```python
from build123d import *

# Parameters (mm, degrees)
ESQUISSE3_W                  = 50
ESQUISSE3_H                  = 43
BOSS_EXTRU_1_DEPTH           = 9
ESQUISSE4_R                  = 2.5
ENL_V_MAT_EXTRU_1_DEPTH      = 1
ENL_V_MAT_EXTRU_1_DEPTH_BACK = 10


with BuildPart() as part:
    # Esquisse3 → Boss.-Extru.1 (new body)
    with BuildSketch(Plane.XY):
        with Locations((25, 21.5)):
            Rectangle(ESQUISSE3_W, ESQUISSE3_H)
    extrude(amount=BOSS_EXTRU_1_DEPTH)

    # Esquisse4 → Enlèv. mat.-Extru.1 (cut, two sides)
    with BuildSketch(Plane.XY.offset(9)) as enl_v_mat_extru_1_sk:
        with Locations((25, 21.5)):
            Circle(ESQUISSE4_R)
    extrude(amount=ENL_V_MAT_EXTRU_1_DEPTH, mode=Mode.SUBTRACT)
    extrude(enl_v_mat_extru_1_sk.sketch, amount=-ENL_V_MAT_EXTRU_1_DEPTH_BACK, mode=Mode.SUBTRACT)


solid = part.part
```
Geometry check sheet. Reference: the model listing, model coordinates, mm. Coordinates: 2 decimals unless noted, no trailing zeros. Order: outer loops, then holes, each group sorted by start corner. A loop starts at its lowest first (then second) coordinate and runs counter-clockwise, first axis right, second up.
Item 1: Mould release check, pull along Y, two halves, no side actions. Record for faces 1 (the cylindrical face through (25, 24, 5)), 2 (the flat face through (25, 43, 4)), 3 (the flat face through (25, 0, 4)), 4 (the flat face through (25, 27, 0)): released by +Y, released by -Y, zero draft, split by the parting line, or undercut.
Item 2: Section check A-A (y = 21.5). Enter the section's corners in (x, z), plus the area to 3 significant figures.
Item 3: Section check B-B (x = 25). Enter the section's corners in (y, z), plus the area to 3 significant figures.
Item 4: Scan lines: line 1 along Y through (x, z) = (25, 3); line 2 along Y through (x, z) = (23.5, 8). Record each from-to range of solid material in increasing order.
Check sheet entries:
1. face 1: undercut
1. face 2: released by +Y
1. face 3: released by -Y
1. face 4: zero draft
2. outline: (0, 0) - (22.5, 0) - (22.5, 9) - (0, 9) - close; (27.5, 0) - (50, 0) - (50, 9) - (27.5, 9) - close
2. area: 405 mm2
3. outline: (0, 0) - (19, 0) - (19, 9) - (0, 9) - close; (24, 0) - (43, 0) - (43, 9) - (24, 9) - close
3. area: 342 mm2
4. line 1: y = 0 to 19, 24 to 43
4. line 2: y = 0 to 19.5, 23.5 to 43
